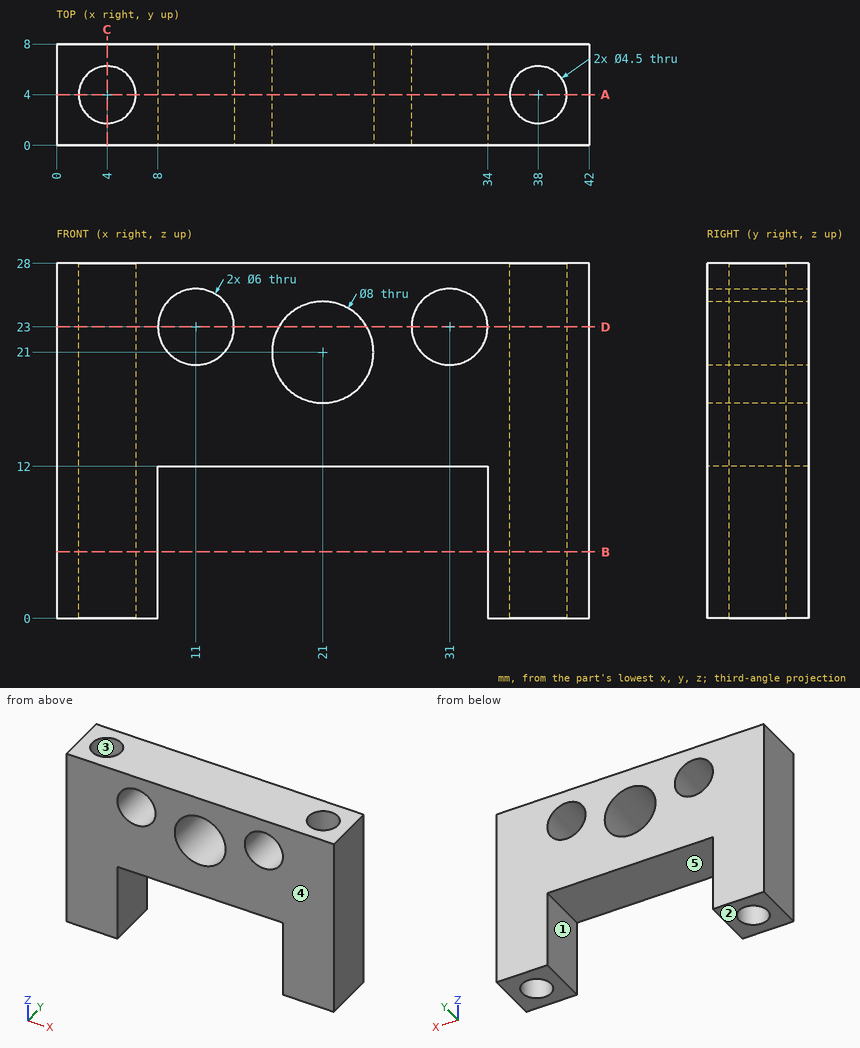
Source: three-view drawing plus pictorial views. Frame: mm from the lowest corner of the part. A direction names the side the tool comes from. Round coordinates to 2 decimals unless told otherwise and drop trailing zeros. Write each loop counter-clockwise with the first axis right and the second up, starting at its lowest first coordinate (ties: lowest second). Pieces come first, ordered by that corner, then holes. Notation, with made-up numbers: M 77,82 L 110,82 A20 cw 110,119 Z; hole C 33.25,27 d10. An arc over 180 degrees is marked long. Use CSV: the item, a comma, the result in double quotes. Start each with the question number.
Q1. Pull-direction query (Y, two-part tool) for the marked faces 3, 4 and 5; classes: +Y half, -Y half, draft (parallel to the pull), parting line (faces both ways), or undercut.
Q2. Cut plane A-A on y = 4. Output: boundary loops of the cut face in (x, z).
Q3. Cut plane C-C on x = 4. Output: boundary loops of the cut face in (y, z).
Q4. Access query for the marked faces 1 and 2. Directions: +Z, -Z, +X, -X, +Y, -Y. A direction counts if a zero-diameter tool reaches every point of the face in a straight line with its end or side. Return the directions, or none.
Q5. Line query: line 1 (Y direction, x = 38, z = 15.5); line 2 (X direction, y = 3.75, z = 3.5); line 3 (X direction, y = 5, z = 18). Output: solid intervals per line, ascending. Write a range as from..to.
Q6. Cut plane B-B on z = 5.25. Output: boundary loops of the cut face in (x, y).
Q7. Cut plane D-D on z = 23. Output: boundary loops of the cut face in (x, y).
Results found:
1,face 3,"undercut"
1,face 4,"-Y half"
1,face 5,"draft"
2,outline,"M 0,0 L 1.75,0 L 1.75,28 L 0,28 Z; M 6.25,0 L 8,0 L 8,12 L 34,12 L 34,0 L 35.75,0 L 35.75,28 L 6.25,28 Z; M 40.25,0 L 42,0 L 42,28 L 40.25,28 Z; hole C 11,23 d6; hole C 21,21 d8; hole C 31,23 d6"
3,outline,"M 0,0 L 1.75,0 L 1.75,28 L 0,28 Z; M 6.25,0 L 8,0 L 8,28 L 6.25,28 Z"
4,face 1,"-Z, +Y, -Y"
4,face 2,"-Z, +X, -X, +Y, -Y"
5,line 1,"0..1.75, 6.25..8"
5,line 2,"0..1.76, 6.24..8, 34..35.76, 40.24..42"
5,line 3,"0..1.98, 6.02..18.35, 23.65..35.98, 40.02..42"
6,outline,"M 0,0 L 8,0 L 8,8 L 0,8 Z; M 34,0 L 42,0 L 42,8 L 34,8 Z; hole C 4,4 d4.5; hole C 38,4 d4.5"
7,outline,"M 0,0 L 8,0 L 8,8 L 0,8 Z; M 14,0 L 17.54,0 L 17.54,8 L 14,8 Z; M 24.46,0 L 28,0 L 28,8 L 24.46,8 Z; M 34,0 L 42,0 L 42,8 L 34,8 Z; hole C 4,4 d4.5; hole C 38,4 d4.5"
